Check sheet for the modelled part. Datum: model origin and axes. Units: mm. A direction names the side the tool comes from. Round coordinates to 2 decimals unless told otherwise and drop trailing zeros. Write each loop counter-clockwise with the first axis right and the second up, starting at its lowest first coordinate (ties: lowest second). Pieces come first, ordered by that corner, then holes. Notation, with made-up numbers: (-29, 40.5) - (27, 40.5) arc R30 ccw to (27, 65.5) - close; hole circle Ø1 at (70.25, 7.5). An arc over 180 degrees is marked (long way). Answer as a JSON object with one key per item and string values. Group by question number.
Item 1: Thickness scan on line 1 (X direction, y = 51, z = -0.5); line 2 (X direction, y = 73, z = 0); line 3 (Y direction, x = -1.5, z = -7.75). Record the ranges inside material, lowest first.
Item 2: Sectioned sample at B-B on y = 54. Record the boundary of the cut face in (x, z), plus the area to 3 significant figures.
Item 3: Release check for a two-part mould opening along X. For faces 1 (the cylindrical face through (-10.074, 75.133, 1.323)), 2 (the flat face through (0, 70.458, -9)), 3 (the flat face through (-8, 0, -1)) record: pulls with the +X half, pulls with the -X half, needs draft (parallel to the pull), parting line crosses it, or undercut.
Item 4: Gauge pin test, flat ends, axial feed: P1, Ø8, axis at y = 71, z = -8, coming from the -X side; P2, Ø5, axis at x = 7.5, y = 116, coming from the -Z side; P3, Ø3, axis at x = 7.5, z = 6, coming from the -Y side; P4, Ø1.5, axis at y = 41, z = 4.5, coming from the -X side. Record the tip position at first contact, or that the pin passes through.
Item 5: Sectioned sample at C-C on y = 75. Record the boundary of the cut face in (x, z).
Item 6: Set-up check for faces 4 (the flat face through (-8, 152.4, -1)), 5 (the flat face through (0, 45.058, -9)): record each of +Z, -Z, +X, -X, +Y, -Y from which the full face is reachable in a straight line by a thin tool's end or side.
Item 7: Sectioned sample at A-A on z = 0. Record the boundary of the cut face in (x, y), plus the area to 3 significant figures.
```python
from build123d import *

# Parameters (mm, degrees)
SKETCH2_R               = 10.16
SKETCH2_R_2             = 7.62
BOSS_EXTRUDE1_DEPTH     = 152.4
CUT_EXTRUDE1_DEPTH      = 154.075834801
CUT_EXTRUDE1_DEPTH_BACK = 154.075834801
SKETCH3_R               = 1
SKETCH4_W               = 5.08
SKETCH4_H               = 25.4
CUT_EXTRUDE2_DEPTH      = 154.075834914


with BuildPart() as part:
    # Sketch2 → Boss-Extrude1 (new body)
    with BuildSketch(Plane(origin=(0, 0, 0), x_dir=(1, 0, 0), z_dir=(0, 1, 0))):
        with Locations(Location((0, 0, 0), (0, 0, 90))):
            Circle(SKETCH2_R)
        with Locations(Location((0, 0, 0), (0, 0, 90))):
            Circle(SKETCH2_R_2, mode=Mode.SUBTRACT)
    extrude(amount=BOSS_EXTRUDE1_DEPTH)

    # Sketch3 → Cut-Extrude1 (cut, two sides: drawn at the far end of the back side and taken through both)
    with BuildSketch(Plane.XY.offset(-CUT_EXTRUDE1_DEPTH_BACK)):
        with Locations((0, 138.43)):
            Circle(SKETCH3_R)
    extrude(amount=CUT_EXTRUDE1_DEPTH + CUT_EXTRUDE1_DEPTH_BACK, mode=Mode.SUBTRACT)

    # Sketch4 → Cut-Extrude2 (cut, through all)
    with BuildSketch(Plane.XY):
        with Locations((0, 57.757755026)):
            Rectangle(SKETCH4_W, SKETCH4_H)
    extrude(amount=-CUT_EXTRUDE2_DEPTH, mode=Mode.SUBTRACT)


solid = part.part
```
Completed:
{
 "1": {"line 1": "-10.15 to -7.6, 7.6 to 10.15", "line 2": "-10.16 to -7.62, 7.62 to 10.16", "line 3": "0 to 45.06, 70.46 to 152.4"},
 "2": {"outline": "(-2.54, -9.84) - (-2.54, -7.18) arc R7.62 cw (long way) to (2.54, -7.18) - (2.54, -9.84) arc R10.16 ccw (long way) to start", "area": "129 mm²"},
 "3": {"face 1": "parting line crosses it", "face 2": "undercut", "face 3": "needs draft"},
 "4": {"P1": "x = -9.34", "P2": "z = -8.84", "P3": "y = 0", "P4": "x = -9.44"},
 "5": {"outline": "circle Ø20.32 at (0, 0); hole circle Ø15.24 at (0, 0)"},
 "6": {"face 4": "+Z, -Z, +X, -X, +Y", "face 5": "-Z"},
 "7": {"outline": "(-10.16, 0) - (-7.62, 0) - (-7.62, 152.4) - (-10.16, 152.4) - close; (7.62, 0) - (10.16, 0) - (10.16, 152.4) - (7.62, 152.4) - close", "area": "774 mm²"}
}
